Read the model definition and answer for the solid it produces. Units are mm, in the model's axes. Coordinates: 2 decimals unless noted, no trailing zeros. Write each loop counter-clockwise with the first axis right and the second up, starting at its lowest first coordinate (ties: lowest second). Pieces come first, ordered by that corner, then holes.
Item 1: Straight lines are drawn through the part: probe 1 along Y at (x, z) = (0, 0.55); probe 2 along X at (y, z) = (-8, 0.2); probe 3 along X at (y, z) = (-12, 1.4). For each, find the intervals that lie inside material, in ascending order.
Item 2: Section C-C (x = 0) is taken. Give the vertices of the cut face in (y, z), then the cut area to 3 significant figures.
Item 3: Determine the mould class of faces 1 (the face through (-4.5, 0, 1)), 2 (the face through (-0.13, -10.76, 0.59)), 3 (the face through (-5, 0, 0)), 4 (the face through (7.9, -13, 0.6)) for opening direction Y: released by +Y, released by -Y, zero draft, split by the parting line, or undercut.
Item 4: Section B-B (y = -5.5) is taken. Give the vertices of the cut face in (x, z), then the cut area to 3 significant figures.
Item 5: Section A-A (x = -2) is taken. Give the vertices of the cut face in (y, z), then the cut area to 3 significant figures.
Item 6: Section D-D (z = 0.8) is taken. Give the vertices of the cut face in (x, y), then the cut area to 3 significant figures.
from build123d import *

# Parameters (mm, degrees)
F0_W     = 20
F0_H     = 30
F0_R     = 1
F0_W_2   = 9
F0_H_2   = 20
F1_DEPTH = 1.5
F2_R     = 7
F3_SIZE  = 0.3


with BuildPart() as f1:
    # F0 (on Top) → F1 (new body)
    with BuildSketch(Plane.XY):
        Rectangle(F0_W, F0_H)
        with Locations((0, -11.75)):
            Circle(F0_R, mode=Mode.SUBTRACT)
        Rectangle(F0_W_2, F0_H_2, mode=Mode.SUBTRACT)
        with Locations((0, 11.75)):
            Circle(F0_R, mode=Mode.SUBTRACT)
    extrude(amount=F1_DEPTH)

    # F2
    f2_edges = [f1.edges().sort_by_distance(p)[0] for p in [
        (-10, -15, 0.75),
        (10, -15, 0.75),
        (10, 15, 0.75),
        (-10, 15, 0.75),
    ]]
    fillet(f2_edges, radius=F2_R)

    # F3
    f3_edges = [f1.edges().sort_by_distance(p)[0] for p in [
        (-1, -11.75, 1.5),
        (-1, 11.75, 1.5),
        (0, 10, 1.5),
        (-4.5, 0, 1.5),
        (0, -10, 1.5),
        (4.5, 0, 1.5),
        (0, 15, 1.5),
        (-7.949747, 12.949747, 1.5),
        (-10, 0, 1.5),
        (7.949747, 12.949747, 1.5),
        (10, 0, 1.5),
        (7.949747, -12.949747, 1.5),
        (0, -15, 1.5),
        (-7.949747, -12.949747, 1.5),
    ]]
    chamfer(f3_edges, length=F3_SIZE)


solid = f1.part
Established:
1. probe 1: y = -15 to -12.75, -10.75 to -10, 10 to 10.75, 12.75 to 15
1. probe 2: x = -10 to -4.5, 4.5 to 10
1. probe 3: x = -8.5 to -1.17, 1.17 to 8.5
2. outline: (-15, 0) - (-12.75, 0) - (-12.75, 1.2) - (-13.05, 1.5) - (-14.7, 1.5) - (-15, 1.2) - close; (-10.75, 0) - (-10, 0) - (-10, 1.2) - (-10.3, 1.5) - (-10.45, 1.5) - (-10.75, 1.2) - close; (10, 0) - (10.75, 0) - (10.75, 1.2) - (10.45, 1.5) - (10.3, 1.5) - (10, 1.2) - close; (12.75, 0) - (15, 0) - (15, 1.2) - (14.7, 1.5) - (13.05, 1.5) - (12.75, 1.2) - close
2. area: 8.64 mm2
3. face 1: undercut
3. face 2: undercut
3. face 3: zero draft
3. face 4: released by -Y
4. outline: (-10, 0) - (-4.5, 0) - (-4.5, 1.2) - (-4.8, 1.5) - (-9.7, 1.5) - (-10, 1.2) - close; (4.5, 0) - (10, 0) - (10, 1.2) - (9.7, 1.5) - (4.8, 1.5) - (4.5, 1.2) - close
4. area: 16.3 mm2
5. outline: (-15, 0) - (-10, 0) - (-10, 1.2) - (-10.3, 1.5) - (-14.7, 1.5) - (-15, 1.2) - close; (10, 0) - (15, 0) - (15, 1.2) - (14.7, 1.5) - (10.3, 1.5) - (10, 1.2) - close
5. area: 14.8 mm2
6. outline: (-10, -8) arc R7 ccw to (-3, -15) - (3, -15) arc R7 ccw to (10, -8) - (10, 8) arc R7 ccw to (3, 15) - (-3, 15) arc R7 ccw to (-10, 8) - close; hole (-4.5, -10) - (4.5, -10) - (4.5, 10) - (-4.5, 10) - close; hole circle Ø2 at (0, -11.75); hole circle Ø2 at (0, 11.75)
6. area: 372 mm2
